The model under review builds one solid part; all positions refer to its coordinate system, in mm. A direction names the side the tool comes from. Coordinates: 2 decimals unless noted, no trailing zeros. Write each loop counter-clockwise with the first axis right and the second up, starting at its lowest first coordinate (ties: lowest second). Pieces come first, ordered by that corner, then holes. Notation, with made-up numbers: (-38.5, -33.75) - (-27.5, -33.75) arc R20 ccw to (-27.5, -8.75) - close; hole circle Ø9 at (34.25, -6). An arc over 180 degrees is marked (long way). Put each result on its own line as item: value.
from build123d import *

# Parameters (mm, degrees)
BOSS_EXTRU_1_DEPTH      = 5
ESQUISSE5_R             = 1.5
ENL_V_MAT_EXTRU_1_DEPTH = 15
BOSS_EXTRU_2_DEPTH      = 63


with BuildPart() as part:
    # Esquisse1 → Boss.-Extru.1 (new body)
    with BuildSketch(Plane.XY):
        Polygon((63, 35), (58, 35), (58, 25), (63, 25), (63, 0), (53, 0), (53, 5), (10, 5), (10, 0), (0, 0), (0, 55), (10, 55), (10, 60), (63, 60), align=None)
    extrude(amount=BOSS_EXTRU_1_DEPTH)

    # Esquisse5 → Enlèv. mat.-Extru.1 (cut)
    with BuildSketch(Plane.ZY):
        with Locations((2.5, 2.5)):
            Circle(ESQUISSE5_R)
        with Locations((2.5, 57.5)):
            Circle(ESQUISSE5_R)
    extrude(amount=-ENL_V_MAT_EXTRU_1_DEPTH, mode=Mode.SUBTRACT)

    # Esquisse8 → Boss.-Extru.2 (add)
    with BuildSketch(Plane(origin=(63, 0, 0), x_dir=(0, 0, -1), z_dir=(1, 0, 0))):
        Polygon((-5, 52), (-9.3, 52), (-9.3, 55.7), (-13, 55.7), (-13, 48), (-5, 48), align=None)
        Polygon((-5, 12), (-5, 8), (-9.3, 8), (-9.3, 4.3), (-13, 4.3), (-13, 12), align=None)
    extrude(amount=-BOSS_EXTRU_2_DEPTH)


solid = part.part
1. To check wall thickness, follow probe 1 along Y at (x, z) = (8.5, 11.25); probe 2 along Y at (x, z) = (11.3, 2.5); probe 3 along Z at (x, y) = (48.5, 13). State the ranges of each line that lie inside material, in increasing order.
Determined:
probe 1: y = 4.3 to 12, 48 to 55.7
probe 2: y = 5 to 56, 59 to 60
probe 3: z = 0 to 5
2. Consider section B-B on y = 2.5. State the section outline as (x, z) points, plus the area to 3 significant figures.
Determined:
outline: (0, 0) - (10, 0) - (10, 1) - (0, 1) - close; (0, 4) - (10, 4) - (10, 5) - (0, 5) - close; (53, 0) - (63, 0) - (63, 5) - (53, 5) - close
area: 70.0 mm^2
3. Consider section D-D on y = 57.5. State the section outline as (x, z) points.
Determined:
outline: (10, 0) - (63, 0) - (63, 5) - (10, 5) - (10, 4) - (15, 4) - (15, 1) - (10, 1) - close
4. For pin 1 Ø1.5 at (y, z) = (57, 3) entering from -X; pin 2 Ø6.5 at (x, z) = (29.5, 8.5) entering from +Y; pin 3 Ø2.5 at (y, z) = (58, 2) entering from -X, all flat-tipped, find the tip position at first contact; note any pin that passes through.
Determined:
pin 1: stops at x = 15
pin 2: stops at y = 55.7
pin 3: stops at x = 10
5. Machinability: for faces 5 (the flat face through (32, 8, 7)), 6 (the cylindrical face through (12.465, 58.987, 2.305)), 7 (the flat face through (61, 35, 2)), which of the approach directions +Z, -Z, +X, -X, +Y, -Y give a long, thin tool a straight path to every point of the face, cutting with its end or side? Answer none if there is none.
Determined:
face 5: +X, -X, -Y
face 6: -X
face 7: +Z, -Z, +X
6. Consider section C-C on x = 27.5. State the section outline as (y, z) points.
Determined:
outline: (4.3, 9.3) - (8, 9.3) - (8, 5) - (5, 5) - (5, 0) - (60, 0) - (60, 5) - (52, 5) - (52, 9.3) - (55.7, 9.3) - (55.7, 13) - (48, 13) - (48, 5) - (12, 5) - (12, 13) - (4.3, 13) - close
7. The part is to be moulded in two halves that separate along X. For faces 1 (the flat face through (32, 48, 9)), 2 (the flat face through (32, 5, 2)), 3 (the flat face through (53, 2, 2)), 4 (the flat face through (63, 48, 4)), say which applies: +X half, -X half, draft (parallel to the pull), parting line (faces both ways), or undercut.
Determined:
face 1: draft
face 2: undercut
face 3: undercut
face 4: +X half
8. Consider section A-A on z = 2.5. State the section outline as (x, y) points.
Determined:
outline: (0, 0) - (10, 0) - (10, 1) - (0, 1) - close; (0, 4) - (10, 4) - (10, 5) - (53, 5) - (53, 0) - (63, 0) - (63, 25) - (58, 25) - (58, 35) - (63, 35) - (63, 60) - (10, 60) - (10, 59) - (15, 59) - (15, 56) - (10, 56) - (10, 55) - (0, 55) - close
